Autodesk Inventor part; units mm, degrees
ref_plane "YZ Plane" through (0, 0, 0) normal (1, 0, 0) x (0, 1, 0)
ref_plane "XZ Plane" through (0, 0, 0) normal (0, 1, 0) x (-1, 0, 0)
ref_plane "XY Plane" through (0, 0, 0) normal (0, 0, 1) x (1, 0, 0)
sketch "Sketch3" plane through (0, 0, 0) normal (0, 1, 0) x (-1, 0, 0)
  line L0 (0, 0) -> (5, 0)
  line L1 (5, 0) -> (-5, 0)
  line L2 (-5, 0) -> (-5, -25)
  line L3 (-5, 0) -> (20, 0) construction
  line L4 (-5, -25) -> (-10, -25)
  line L5 (-10, -25) -> (-10, 5)
  line L6 (-10, 5) -> (0, 5)
  line L7 (0, 5) -> (5, 5)
  line L8 (5, 5) -> (5, 0)
  line L9 (5, 0) -> (5, -25)
  line L10 (5, -25) -> (10, -25)
  line L11 (10, -25) -> (10, 5)
  line L12 (10, 5) -> (5, 5)
  dimension "d2" = 5
  dimension "d3" = 10
  dimension "d4" = 0
  dimension "d5" = 25
  dimension "d6" = 90
  dimension "d7" = 5
  dimension "d8" = 30
  dimension "d9" = 5
extrude "Extrusion1" add sketch "Sketch3" along normal mid plane 75
sketch "Sketch7" plane through (5, 37.5, 0) normal (0, 0, -1) x (-1, 0, 0)
  line L0 (5, -37.5) -> (10, -37.5) construction
  line L1 (10, -37.5) -> (0, -37.5) construction
  dimension "d25" = 5
  dimension "d26" = 10
properties part number "TSU_Middle_Clamp"
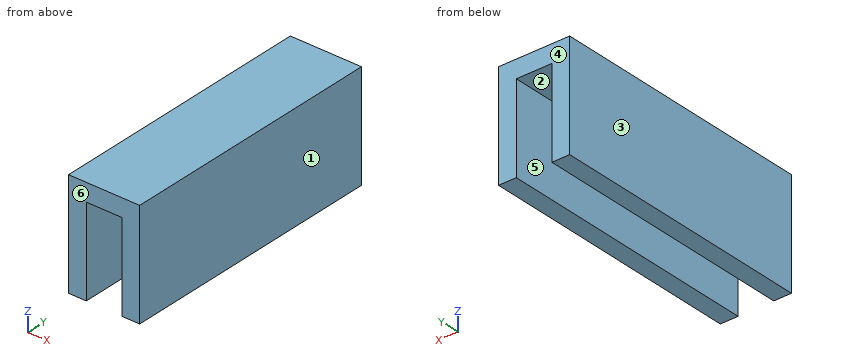
Work out the finished part from the listing and answer in its coordinate system (mm). Face numbers are marked on the shaded views. A direction names the side the tool comes from. Round coordinates to 2 decimals unless told otherwise and drop trailing zeros. Loops run counter-clockwise (first coordinate to the right, second up) from the corner with the lowest first, then second, coordinate; pieces in that order, holes last. Notation, with made-up numbers: (21, -39.5) -> (25, -39.5) arc R30 cw to (25, -9.5) -> close; hole circle Ø8 at (51.25, 24.25). An arc over 180 degrees is marked (long way). Write each question's results on one line, items separated by ' | '. Start each with the question number.
1. Section A-A (z = -1.5) is taken. Determine the outline of the cut face in (x, y).
2. Section B-B (y = -30) is taken. Determine the outline of the cut face in (x, z).
3. Section C-C (x = -2.75) is taken. Determine the outline of the cut face in (y, z).
4. A tool of negligible diameter and unlimited length cuts with its end or side. For the marked faces 5 and 6, from which of +Z, -Z, +X, -X, +Y, -Y can it reach the whole face along a straight path? Write none if from no direction.
5. Find the intervals of material crossed by probe 1 along X at (y, z) = (22, -22.5); probe 2 along Z at (x, y) = (4.5, -19.5), in increasing order. Write a range as from..to.
6. Given pin 1 Ø2 at (x, y) = (2.5, 16) entering from -Z, flat-ended and moving along its own axis, determine where the tip first touches the part or whether it passes through.
7. For a pull along X with two mould halves and no side action, classify the marked faces 1, 2, 3 and 4 as +X half, -X half, draft (parallel to the pull), parting line (faces both ways), or undercut.
Evaluation:
1) outline: (-10, -37.5) -> (-5, -37.5) -> (-5, 37.5) -> (-10, 37.5) -> close; (5, -37.5) -> (10, -37.5) -> (10, 37.5) -> (5, 37.5) -> close
2) outline: (-10, -25) -> (-5, -25) -> (-5, 0) -> (5, 0) -> (5, -25) -> (10, -25) -> (10, 5) -> (-10, 5) -> close
3) outline: (-37.5, 0) -> (37.5, 0) -> (37.5, 5) -> (-37.5, 5) -> close
4) face 5: -Z, +Y, -Y | face 6: +Z, -Z, +X, -X, -Y
5) probe 1: x = -10..-5, 5..10 | probe 2: z = 0..5
6) pin 1: stops at z = 0
7) face 1: +X half | face 2: undercut | face 3: -X half | face 4: draft
